Could you check a few things on this drawing? It's one solid part, dimensions in mm from its lowest x, y, z. Coordinates: 2 decimals unless noted, no trailing zeros. Loops run counter-clockwise (first coordinate to the right, second up) from the corner with the lowest first, then second, coordinate; pieces in that order, holes last.
1) Imagine slicing it at D-D on x = 19. Please give me the cut outline in (y, z), plus the area to 3 significant figures.
2) Imagine slicing it at C-C on z = 2.75. Please give me the cut outline in (x, y) (3 decimals), plus the area to 3 significant figures.
3) Imagine slicing it at B-B on y = 26. Please give me the cut outline in (x, z) (3 decimals), plus the area to 3 significant figures.
4) If I drill on line 1 along X through (y, z) = (27, 5) (3 decimals); line 2 along Y through (x, z) = (65, 19.5); line 3 along Z through (x, y) = (50, 8.5), over which ranges is the centre line in solid material (lowest first)?
5) Imagine slicing it at A-A on z = 15.75. Please give me the cut outline in (x, y) (3 decimals).
6) Will these pins go through, and if not, where does the flat tip stop? P1, Ø8, axis at x = 17.5, y = 19.5, coming from the -Z side; P2, Ø12.5, axis at x = 65, z = 18.5, coming from the -Y side; P3, Ø4, axis at y = 14, z = 1, coming from the +X side (3 decimals); P4, Ø13.5, axis at x = 34.5, y = 16, coming from the +Z side.
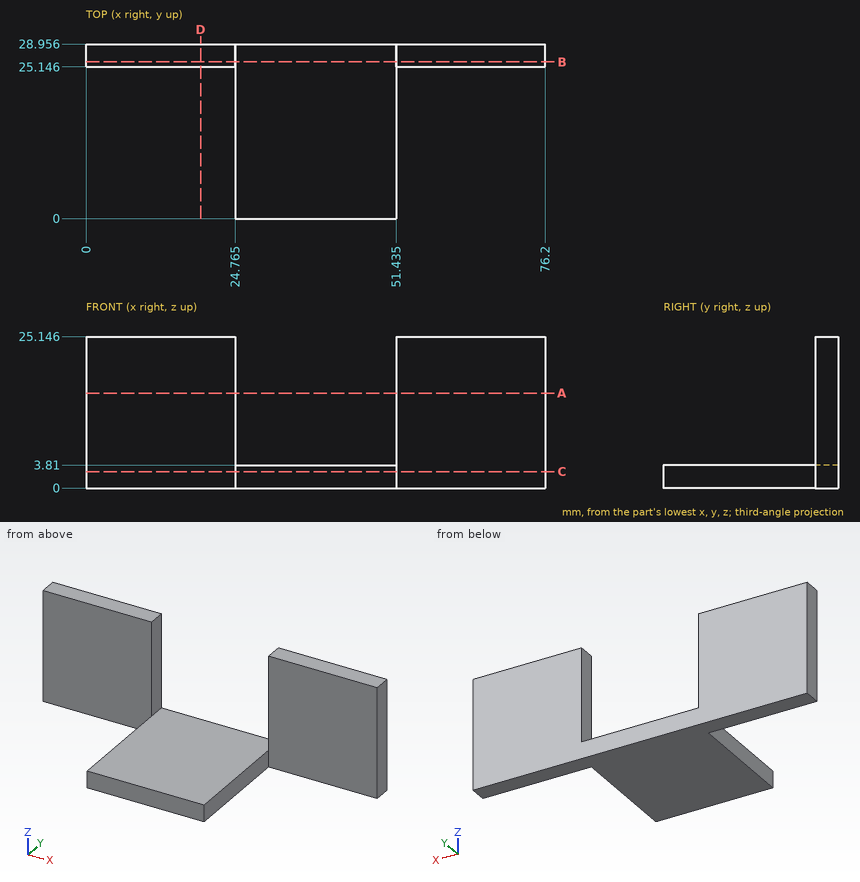
Filled in:
1. outline: (25.15, 0) - (28.96, 0) - (28.96, 25.15) - (25.15, 25.15) - close
1. area: 95.8 mm2
2. outline: (0, 25.146) - (24.765, 25.146) - (24.765, 0) - (51.435, 0) - (51.435, 25.146) - (76.2, 25.146) - (76.2, 28.956) - (0, 28.956) - close
2. area: 961 mm2
3. outline: (0, 0) - (76.2, 0) - (76.2, 25.146) - (51.435, 25.146) - (51.435, 3.81) - (24.765, 3.81) - (24.765, 25.146) - (0, 25.146) - close
3. area: 1,350 mm2
4. line 1: x = 0 to 24.765, 51.435 to 76.2
4. line 2: y = 25.15 to 28.96
4. line 3: z = 0 to 3.81
5. outline: (0, 25.146) - (24.765, 25.146) - (24.765, 28.956) - (0, 28.956) - close; (51.435, 25.146) - (76.2, 25.146) - (76.2, 28.956) - (51.435, 28.956) - close
6. P1: passes through
6. P2: stops at y = 25.15
6. P3: stops at x = 51.435
6. P4: stops at z = 3.81
